Here's how the part is built. I have some questions about the finished solid (model axes, mm). Round coordinates to 2 decimals unless told otherwise and drop trailing zeros. Order: outer loops, then holes, each group sorted by start corner. A loop starts at its lowest first (then second) coordinate and runs counter-clockwise, first axis right, second up. Notation, with made-up numbers: (-8, -34) - (9, -34) arc R23 cw to (9, -8) - close; hole circle Ø7 at (60.25, 25). An arc over 180 degrees is marked (long way). One line per item, written item: value.
from build123d import *

# Parameters (mm, degrees)
SKETCH1_W           = 400
SKETCH1_H           = 696
BOSS_EXTRUDE1_DEPTH = 18
SKETCH2_W           = 400
SKETCH2_H           = 9
CUT_EXTRUDE1_DEPTH  = 9
SKETCH3_W           = 400
SKETCH3_H           = 18
CUT_EXTRUDE2_DEPTH  = 9


with BuildPart() as part:
    # Sketch1 → Boss-Extrude1 (new body)
    with BuildSketch(Plane(origin=(0, 0, 0), x_dir=(0, 0, -1), z_dir=(1, 0, 0))):
        Rectangle(SKETCH1_W, SKETCH1_H)
    extrude(amount=BOSS_EXTRUDE1_DEPTH)

    # Sketch2 → Cut-Extrude1 (cut)
    with BuildSketch(Plane.ZY):
        with Locations((0, -343.5)):
            Rectangle(SKETCH2_W, SKETCH2_H)
        with Locations((0, 343.5)):
            Rectangle(SKETCH2_W, SKETCH2_H)
    extrude(amount=-CUT_EXTRUDE1_DEPTH, mode=Mode.SUBTRACT)

    # Sketch3 → Cut-Extrude2 (cut)
    with BuildSketch(Plane.ZY):
        Rectangle(SKETCH3_W, SKETCH3_H)
    extrude(amount=-CUT_EXTRUDE2_DEPTH, mode=Mode.SUBTRACT)


solid = part.part
Q1. We'd pull the mould along Y, two halves only. Please class faces 1 (the flat face through (0, -172, 3)), 2 (the flat face through (9, 0, -3)): released by +Y, released by -Y, zero draft, split by the parting line, or undercut.
Results list:
face 1: zero draft
face 2: undercut
Q2. If we section it at A-A, the plane x = 3.75: Please give me the cut outline in (y, z), then the cut area to 3 significant figures.
Results list:
outline: (-339, -200) - (-9, -200) - (-9, 200) - (-339, 200) - close; (9, -200) - (339, -200) - (339, 200) - (9, 200) - close
area: 264,000 mm²
Q3. If we section it at B-B, the plane z = -171: Please give me the cut outline in (x, y), then the cut area to 3 significant figures.
Results list:
outline: (0, -339) - (9, -339) - (9, -348) - (18, -348) - (18, 348) - (9, 348) - (9, 339) - (0, 339) - (0, 9) - (9, 9) - (9, -9) - (0, -9) - close
area: 12,200 mm²
Q4. If I drill on line 1 along Y through (x, z) = (1, -85.5); line 2 along X through (y, z) = (-5.5, -28), over which ranges is the centre line in solid material (lowest first)?
Results list:
line 1: -339 to -9, 9 to 339
line 2: 9 to 18
Q5. Will these pins go through, and if not, where does the flat tip stop? pin 1 (5.5 mm diameter, centred on y = -3.5, z = -68, fed in from -X); pin 2 (7 mm diameter, centred on x = 4.5, z = -75.5, fed in from +Y); pin 3 (4.5 mm diameter, centred on x = 2.5, z = -83, fed in from -Y).
Results list:
pin 1: x = 9
pin 2: y = 339
pin 3: y = -339
